Verification items for the finished model (mm, model axes). A direction names the side the tool comes from. Give positions to 0.01 mm unless a question says otherwise; leave off trailing zeros. Write each loop counter-clockwise with the first axis right and the second up, starting at its lowest first coordinate (ties: lowest second). Pieces come first, ordered by that corner, then holes.
from build123d import *

# Parameters (mm, degrees)
CUT_EXTRUDE_1_REACH = 52.931
SKETCH_2_R          = 1.7
SKETCH_2_R_2        = 1.5


with BuildPart() as part:
    # Sketch 1 → Revolve 1 (revolve)
    with BuildSketch(Plane(origin=(0, 0, 0), x_dir=(1, 0, 0), z_dir=(0, 1, 0)), mode=Mode.PRIVATE) as revolve_1_sk:
        Polygon((10, 6), (20, 6), (20, 5), (20.5, 5), (20.5, 6), (35, 6), (35, -6), (20.5, -6), (20.5, -5), (20, -5), (20, -6), (10, -6), align=None)
    revolve(revolve_1_sk.sketch.rotate(Axis((0, 0, -11.223459705), (0, 0, 1)), 180), axis=Axis((0, 0, -11.223459705), (0, 0, 1)))

    # Sketch 2 → Cut-Extrude 1 (cut, up to next)
    with BuildSketch(Plane(origin=(0, 0, -6), x_dir=(-1, 0, 0), z_dir=(0, 0, -1)), mode=Mode.PRIVATE) as cut_extrude_1_sk1:
        with Locations((0, 28.5)):
            Circle(SKETCH_2_R)
    cut_extrude_1_tool1 = extrude(cut_extrude_1_sk1.sketch, amount=-CUT_EXTRUDE_1_REACH, mode=Mode.PRIVATE) & part.part
    # Sketch 2 → Cut-Extrude 1 (cut, up to next)
    with BuildSketch(Plane(origin=(0, 0, -6), x_dir=(-1, 0, 0), z_dir=(0, 0, -1)), mode=Mode.PRIVATE) as cut_extrude_1_sk2:
        with Locations((24.681724008, 14.25)):
            Circle(SKETCH_2_R)
    cut_extrude_1_tool2 = extrude(cut_extrude_1_sk2.sketch, amount=-CUT_EXTRUDE_1_REACH, mode=Mode.PRIVATE) & part.part
    # Sketch 2 → Cut-Extrude 1 (cut, up to next)
    with BuildSketch(Plane(origin=(0, 0, -6), x_dir=(-1, 0, 0), z_dir=(0, 0, -1)), mode=Mode.PRIVATE) as cut_extrude_1_sk3:
        with Locations((24.681724008, -14.25)):
            Circle(SKETCH_2_R)
    cut_extrude_1_tool3 = extrude(cut_extrude_1_sk3.sketch, amount=-CUT_EXTRUDE_1_REACH, mode=Mode.PRIVATE) & part.part
    # Sketch 2 → Cut-Extrude 1 (cut, up to next)
    with BuildSketch(Plane(origin=(0, 0, -6), x_dir=(-1, 0, 0), z_dir=(0, 0, -1)), mode=Mode.PRIVATE) as cut_extrude_1_sk4:
        with Locations((0, -28.5)):
            Circle(SKETCH_2_R)
    cut_extrude_1_tool4 = extrude(cut_extrude_1_sk4.sketch, amount=-CUT_EXTRUDE_1_REACH, mode=Mode.PRIVATE) & part.part
    # Sketch 2 → Cut-Extrude 1 (cut, up to next)
    with BuildSketch(Plane(origin=(0, 0, -6), x_dir=(-1, 0, 0), z_dir=(0, 0, -1)), mode=Mode.PRIVATE) as cut_extrude_1_sk5:
        with Locations((-24.681724008, -14.25)):
            Circle(SKETCH_2_R)
    cut_extrude_1_tool5 = extrude(cut_extrude_1_sk5.sketch, amount=-CUT_EXTRUDE_1_REACH, mode=Mode.PRIVATE) & part.part
    # Sketch 2 → Cut-Extrude 1 (cut, up to next)
    with BuildSketch(Plane(origin=(0, 0, -6), x_dir=(-1, 0, 0), z_dir=(0, 0, -1)), mode=Mode.PRIVATE) as cut_extrude_1_sk6:
        with Locations((-24.681724008, 14.25)):
            Circle(SKETCH_2_R)
    cut_extrude_1_tool6 = extrude(cut_extrude_1_sk6.sketch, amount=-CUT_EXTRUDE_1_REACH, mode=Mode.PRIVATE) & part.part
    # Sketch 2 → Cut-Extrude 1 (cut, up to next)
    with BuildSketch(Plane(origin=(0, 0, -6), x_dir=(-1, 0, 0), z_dir=(0, 0, -1)), mode=Mode.PRIVATE) as cut_extrude_1_sk7:
        with Locations((0, 14)):
            Circle(SKETCH_2_R_2)
    cut_extrude_1_tool7 = extrude(cut_extrude_1_sk7.sketch, amount=-CUT_EXTRUDE_1_REACH, mode=Mode.PRIVATE) & part.part
    # Sketch 2 → Cut-Extrude 1 (cut, up to next)
    with BuildSketch(Plane(origin=(0, 0, -6), x_dir=(-1, 0, 0), z_dir=(0, 0, -1)), mode=Mode.PRIVATE) as cut_extrude_1_sk8:
        with Locations((12.124355653, 7)):
            Circle(SKETCH_2_R_2)
    cut_extrude_1_tool8 = extrude(cut_extrude_1_sk8.sketch, amount=-CUT_EXTRUDE_1_REACH, mode=Mode.PRIVATE) & part.part
    # Sketch 2 → Cut-Extrude 1 (cut, up to next)
    with BuildSketch(Plane(origin=(0, 0, -6), x_dir=(-1, 0, 0), z_dir=(0, 0, -1)), mode=Mode.PRIVATE) as cut_extrude_1_sk9:
        with Locations((12.124355653, -7)):
            Circle(SKETCH_2_R_2)
    cut_extrude_1_tool9 = extrude(cut_extrude_1_sk9.sketch, amount=-CUT_EXTRUDE_1_REACH, mode=Mode.PRIVATE) & part.part
    # Sketch 2 → Cut-Extrude 1 (cut, up to next)
    with BuildSketch(Plane(origin=(0, 0, -6), x_dir=(-1, 0, 0), z_dir=(0, 0, -1)), mode=Mode.PRIVATE) as cut_extrude_1_sk10:
        with Locations((0, -14)):
            Circle(SKETCH_2_R_2)
    cut_extrude_1_tool10 = extrude(cut_extrude_1_sk10.sketch, amount=-CUT_EXTRUDE_1_REACH, mode=Mode.PRIVATE) & part.part
    # Sketch 2 → Cut-Extrude 1 (cut, up to next)
    with BuildSketch(Plane(origin=(0, 0, -6), x_dir=(-1, 0, 0), z_dir=(0, 0, -1)), mode=Mode.PRIVATE) as cut_extrude_1_sk11:
        with Locations((-12.124355653, -7)):
            Circle(SKETCH_2_R_2)
    cut_extrude_1_tool11 = extrude(cut_extrude_1_sk11.sketch, amount=-CUT_EXTRUDE_1_REACH, mode=Mode.PRIVATE) & part.part
    # Sketch 2 → Cut-Extrude 1 (cut, up to next)
    with BuildSketch(Plane(origin=(0, 0, -6), x_dir=(-1, 0, 0), z_dir=(0, 0, -1)), mode=Mode.PRIVATE) as cut_extrude_1_sk12:
        with Locations((-12.124355653, 7)):
            Circle(SKETCH_2_R_2)
    cut_extrude_1_tool12 = extrude(cut_extrude_1_sk12.sketch, amount=-CUT_EXTRUDE_1_REACH, mode=Mode.PRIVATE) & part.part
    add(cut_extrude_1_tool1.solids().sort_by_distance((0, 28.5, -6))[0], mode=Mode.SUBTRACT)
    add(cut_extrude_1_tool2.solids().sort_by_distance((-24.681724, 14.25, -6))[0], mode=Mode.SUBTRACT)
    add(cut_extrude_1_tool3.solids().sort_by_distance((-24.681724, -14.25, -6))[0], mode=Mode.SUBTRACT)
    add(cut_extrude_1_tool4.solids().sort_by_distance((0, -28.5, -6))[0], mode=Mode.SUBTRACT)
    add(cut_extrude_1_tool5.solids().sort_by_distance((24.681724, -14.25, -6))[0], mode=Mode.SUBTRACT)
    add(cut_extrude_1_tool6.solids().sort_by_distance((24.681724, 14.25, -6))[0], mode=Mode.SUBTRACT)
    add(cut_extrude_1_tool7.solids().sort_by_distance((0, 14, -6))[0], mode=Mode.SUBTRACT)
    add(cut_extrude_1_tool8.solids().sort_by_distance((-12.124356, 7, -6))[0], mode=Mode.SUBTRACT)
    add(cut_extrude_1_tool9.solids().sort_by_distance((-12.124356, -7, -6))[0], mode=Mode.SUBTRACT)
    add(cut_extrude_1_tool10.solids().sort_by_distance((0, -14, -6))[0], mode=Mode.SUBTRACT)
    add(cut_extrude_1_tool11.solids().sort_by_distance((12.124356, -7, -6))[0], mode=Mode.SUBTRACT)
    add(cut_extrude_1_tool12.solids().sort_by_distance((12.124356, 7, -6))[0], mode=Mode.SUBTRACT)


solid = part.part
Item 1: Depth check by flat-ended pin: pin 1 (3.5 mm diameter, centred on x = 12.12, y = -7, fed in from +Z); pin 2 (1 mm diameter, centred on y = 17, z = -3, fed in from +X); pin 3 (5 mm diameter, centred on x = 16.5, z = -1.5, fed in from -Y); pin 4 (6 mm diameter, centred on x = 8, z = -2.5, fed in from -Y). Enter the tip coordinate at first touch or a pass-through.
Answer key:
pin 1: stops at z = 6
pin 2: stops at x = 30.87
pin 3: stops at y = -32.08
pin 4: stops at y = -34.64
Item 2: Release check for a two-part mould opening along X. For faces 4 (the face through (-18.937, 7.852, 5.493)), 5 (the face through (-5, -9, -6)), 6 (the face through (7.587, 34.168, 0.084)) record: released by +X, released by -X, zero draft, split by the parting line, or undercut.
Answer key:
face 4: undercut
face 5: zero draft
face 6: split by the parting line
Item 3: Scan lines: line 1 along Y through (x, z) = (0, 3.75); line 2 along X through (y, z) = (-7.5, -2.25); line 3 along X through (y, z) = (-23, 3.5). Record each from-to range of solid material in increasing order.
Answer key:
line 1: y = -35 to -30.2, -26.8 to -15.5, -12.5 to -10, 10 to 12.5, 15.5 to 26.8, 30.2 to 35
line 2: x = -34.19 to -13.54, -10.71 to -6.61, 6.61 to 10.71, 13.54 to 34.19
line 3: x = -26.38 to 26.38
Item 4: Sectioned sample at B-B on y = -28.5. Record the cut outline in (x, z), then the cut area to 3 significant figures.
Answer key:
outline: (-20.32, -6) - (-1.7, -6) - (-1.7, 6) - (-20.32, 6) - close; (1.7, -6) - (20.32, -6) - (20.32, 6) - (1.7, 6) - close
area: 447 mm2
Item 5: Sectioned sample at D-D on x = -6. Record the cut outline in (y, z).
Answer key:
outline: (-34.48, -6) - (-19.6, -6) - (-19.6, -5) - (-19.08, -5) - (-19.08, -6) - (-8, -6) - (-8, 6) - (-19.08, 6) - (-19.08, 5) - (-19.6, 5) - (-19.6, 6) - (-34.48, 6) - close; (8, -6) - (19.08, -6) - (19.08, -5) - (19.6, -5) - (19.6, -6) - (34.48, -6) - (34.48, 6) - (19.6, 6) - (19.6, 5) - (19.08, 5) - (19.08, 6) - (8, 6) - close
Item 6: Sectioned sample at C-C on x = -24. Record the cut outline in (y, z), then the cut area to 3 significant figures.
Answer key:
outline: (-25.48, -6) - (-15.81, -6) - (-15.81, 6) - (-25.48, 6) - close; (-12.69, -6) - (12.69, -6) - (12.69, 6) - (-12.69, 6) - close; (15.81, -6) - (25.48, -6) - (25.48, 6) - (15.81, 6) - close
area: 537 mm2
Item 7: Sectioned sample at A-A on z = -2.75. State how many separate pieces and enclosed holes the cut face has, then the cut area to 3 significant figures.
Answer key:
separate pieces: 1
enclosed holes: 13
area: 3,440 mm2
Item 8: Set-up check for faces 1 (the face through (19.98, -0.88, -5.49)), 2 (the face through (-9, 18.1, 5)), 3 (the face through (11.43, 5.67, -0.08)): record each of +Z, -Z, +X, -X, +Y, -Y from which the full face is reachable in a straight line by a thin tool's end or side.
Answer key:
face 1: -Z
face 2: +Z
face 3: +Z, -Z
